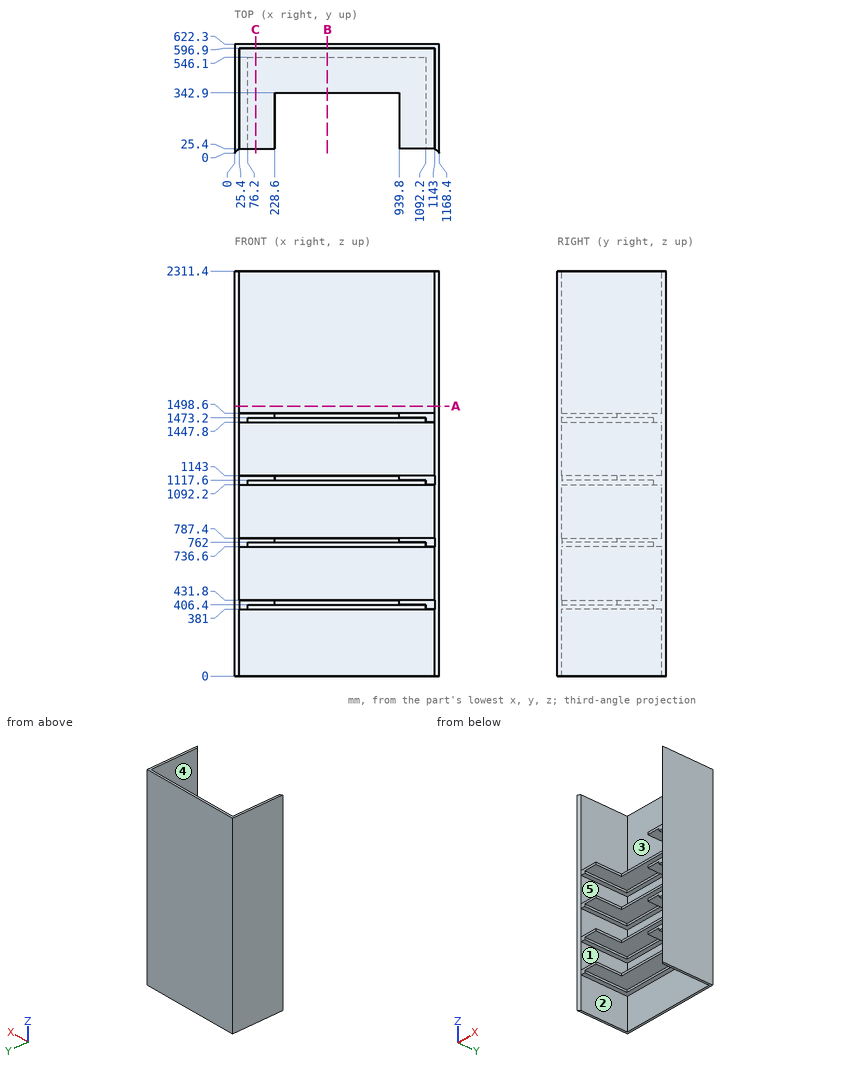
Geometry check sheet. Reference: drawing and pictorial views, mm from the part's lowest x, y, z. A direction names the side the tool comes from. Give positions to 0.01 mm unless a question says otherwise; leave off trailing zeros. Order: outer loops, then holes, each group sorted by start corner. A loop starts at its lowest first (then second) coordinate and runs counter-clockwise, first axis right, second up. Notation, with made-up numbers: M 67.25,51 L 75.25,51 A9 ccw 75.25,60 Z; hole C 49,89.25 d10. An arc over 180 degrees is marked long. Answer in a Markdown table with one row per item. Add a question column.
Item 1: Tool access check on the marked faces 1, 2 and 3. Record the directions out of +Z, -Z, +X, -X, +Y, -Y that give a thin tool (end or side, any length) a straight path to the whole face; none if there is none.
Item 2: Gauge pin test, flat ends, axial feed: pin 1 (1.5 mm diameter, centred on x = 366.5, z = 1580, fed in from -Y); pin 2 (12.5 mm diameter, centred on y = 326.5, z = 390, fed in from -X); pin 3 (15 mm diameter, centred on x = 992, z = 1124, fed in from -Y); pin 4 (20.5 mm diameter, centred on x = 508, z = 415.5, fed in from -Y). Record the tip position at first contact, or that the pin passes through.
Item 3: Scan lines: probe 1 along Z at (x, y) = (1079.5, 316.5); probe 2 along Z at (x, y) = (50, 58.5); probe 3 along X at (y, z) = (289, 1218.5). Record each from-to range of solid material in increasing order. Write a range as from..to.
Item 4: Mould release check, pull along Z, two halves, no side actions. Record for the marked faces 4 and 5: released by +Z, released by -Z, zero draft, split by the parting line, or undercut.
Item 5: Section check C-C, the plane x = 120.5. Enter the section's corners in (y, z), and give its area (3 significant figures).
Item 6: Section check A-A, the plane z = 1540. Enter the section's corners in (x, y), and give its area (3 significant figures).
Item 7: Section check B-B, the plane x = 530. Enter the section's corners in (y, z), and give its area (3 significant figures).
Filled sheet:
| question | item | result |
|---|---|---|
| 1 | face 1 | -Y |
| 1 | face 2 | -Z, -Y |
| 1 | face 3 | +Z, -Y |
| 2 | pin 1 | stops at y = 596.9 |
| 2 | pin 2 | stops at x = 0 |
| 2 | pin 3 | stops at y = 25.4 |
| 2 | pin 4 | stops at y = 342.9 |
| 3 | probe 1 | z = 406.4..431.8, 762..787.4, 1117.6..1143, 1473.2..1498.6 |
| 3 | probe 2 | z = 381..431.8, 736.6..787.4, 1092.2..1143, 1447.8..1498.6 |
| 3 | probe 3 | x = 0..25.4, 1143..1168.4 |
| 4 | face 4 | zero draft |
| 4 | face 5 | undercut |
| 5 | outline | M 25.4,406.4 L 546.1,406.4 L 546.1,381 L 596.9,381 L 596.9,0 L 622.3,0 L 622.3,2311.4 L 596.9,2311.4 L 596.9,1498.6 L 25.4,1498.6 L 25.4,1473.2 L 546.1,1473.2 L 546.1,1447.8 L 596.9,1447.8 L 596.9,1143 L 25.4,1143 L 25.4,1117.6 L 546.1,1117.6 L 546.1,1092.2 L 596.9,1092.2 L 596.9,787.4 L 25.4,787.4 L 25.4,762 L 546.1,762 L 546.1,736.6 L 596.9,736.6 L 596.9,431.8 L 25.4,431.8 Z |
| 5 | area | 122,000 mm^2 |
| 6 | outline | M 0,0 L 25.4,25.4 L 25.4,596.9 L 1143,596.9 L 1143,25.4 L 1168.4,0 L 1168.4,622.3 L 0,622.3 Z |
| 6 | area | 59,400 mm^2 |
| 7 | outline | M 342.9,406.4 L 546.1,406.4 L 546.1,381 L 596.9,381 L 596.9,0 L 622.3,0 L 622.3,2311.4 L 596.9,2311.4 L 596.9,1498.6 L 342.9,1498.6 L 342.9,1473.2 L 546.1,1473.2 L 546.1,1447.8 L 596.9,1447.8 L 596.9,1143 L 342.9,1143 L 342.9,1117.6 L 546.1,1117.6 L 546.1,1092.2 L 596.9,1092.2 L 596.9,787.4 L 342.9,787.4 L 342.9,762 L 546.1,762 L 546.1,736.6 L 596.9,736.6 L 596.9,431.8 L 342.9,431.8 Z |
| 7 | area | 89,700 mm^2 |
